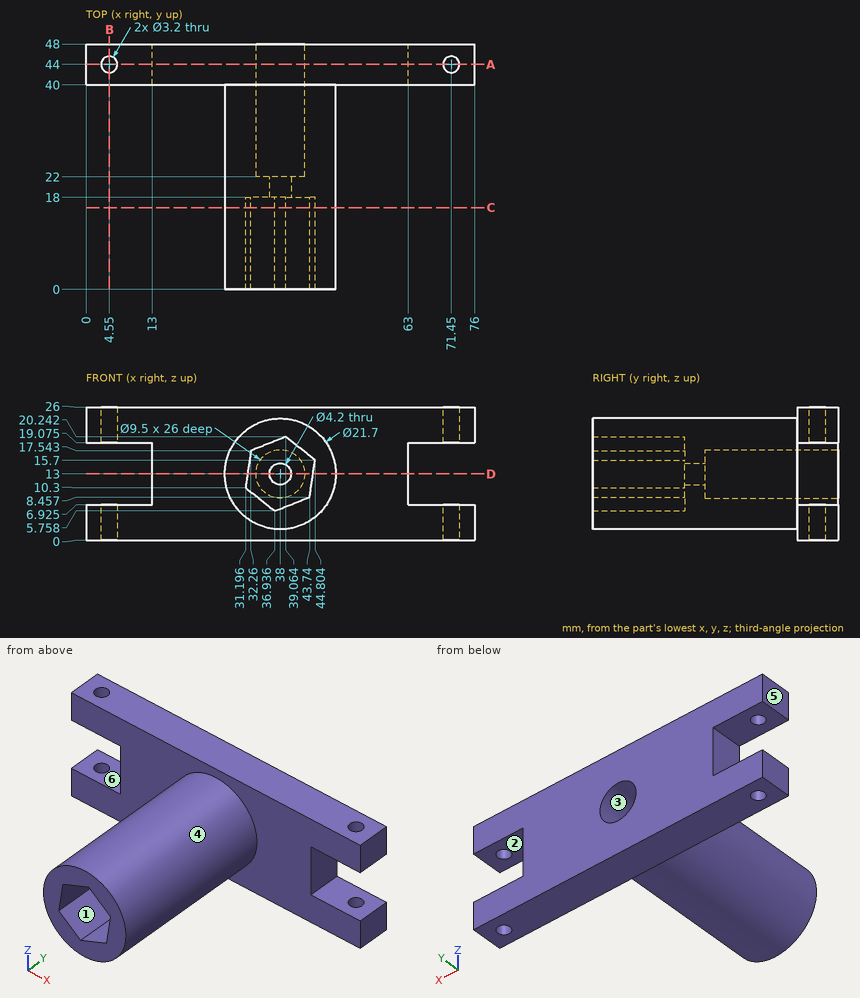
Here's the drawing with two shaded views (mm, measured from the low corner). I have some questions. A direction names the side the tool comes from. Round coordinates to 2 decimals unless told otherwise and drop trailing zeros. Loops run counter-clockwise (first coordinate to the right, second up) from the corner with the lowest first, then second, coordinate; pieces in that order, holes last.
Item 1: Suppose I cut it at A-A, the plane y = 44. State how many separate pieces and enclosed holes the cut face has, then the cut area to 3 significant figures.
Item 2: Suppose I cut it at D-D, the plane z = 13. Write out the boundary of the cut face in (x, y).
Item 3: Will these pins go through, and if not, where does the flat tip stop? pin 1 Ø10 at (x, y) = (56.5, 6.5) entering from +Z; pin 2 Ø6.5 at (x, z) = (38, 13) entering from -Y; pin 3 Ø7.5 at (x, z) = (38, 13) entering from +Y; pin 4 Ø8 at (y, z) = (20, 23) entering from -X.
Item 4: Suppose I cut it at C-C, the plane y = 16. Write out the boundary of the cut face in (x, z).
Item 5: Suppose I cut it at B-B, the plane x = 4.55. Write out the boundary of the cut face in (y, z) (1 decimal).
Item 6: If we mould it in two halves opening along Z, with no side actions, what happens to the marked faces 4, 5 and 6? For each: +Z half, -Z half, draft (parallel to the pull), parting line (faces both ways), or undercut.
Item 7: Which directions (+Z, -Z, +X, -X, +Y, -Y) give clear straight access to the entire face, cutting with the end or side of a thin tool? Please do the marked faces 1, 2 and 3.
Item 8: Please list where these lines run through material, in increasing order: L1, parallel to Z at x = 38, y = 19; L2, parallel to X at y = 30.25, z = 13; L3, parallel to X at y = 41.5, z = 13.
Reported:
1. separate pieces: 5
1. enclosed holes: 1
1. area: 1,500 mm2
2. outline: (13, 40) - (27.15, 40) - (27.15, 0) - (31.59, 0) - (31.59, 18) - (35.9, 18) - (35.9, 22) - (33.25, 22) - (33.25, 48) - (13, 48) - close; (40.1, 18) - (44.41, 18) - (44.41, 0) - (48.85, 0) - (48.85, 40) - (63, 40) - (63, 48) - (42.75, 48) - (42.75, 22) - (40.1, 22) - close
3. pin 1: passes through
3. pin 2: stops at y = 18
3. pin 3: stops at y = 22
3. pin 4: stops at x = 28.96
4. outline: circle Ø21.7 at (38, 13); hole (31.2, 10.3) - (36.94, 5.76) - (43.74, 8.46) - (44.8, 15.7) - (39.06, 20.24) - (32.26, 17.54) - close
5. outline: (40, 0) - (42.4, 0) - (42.4, 6.9) - (40, 6.9) - close; (40, 19.1) - (42.4, 19.1) - (42.4, 26) - (40, 26) - close; (45.6, 0) - (48, 0) - (48, 6.9) - (45.6, 6.9) - close; (45.6, 19.1) - (48, 19.1) - (48, 26) - (45.6, 26) - close
6. face 4: parting line
6. face 5: draft
6. face 6: undercut
7. face 1: -Y
7. face 2: +X, +Y, -Y
7. face 3: +Y
8. L1: z = 2.15 to 10.9, 15.1 to 23.85
8. L2: x = 27.15 to 33.25, 42.75 to 48.85
8. L3: x = 13 to 33.25, 42.75 to 63
